Geometry check sheet. Reference: the model listing, model coordinates, mm. Face numbers are marked on the shaded views. A direction names the side the tool comes from. Round coordinates to 2 decimals unless told otherwise and drop trailing zeros. Order: outer loops, then holes, each group sorted by start corner. A loop starts at its lowest first (then second) coordinate and runs counter-clockwise, first axis right, second up. Notation, with made-up numbers: (3.5, -34.5) - (57.5, -34.5) arc R24 ccw to (57.5, 0.5) - close; hole circle Ø10 at (8, -0.75). An arc over 180 degrees is marked (long way). One line per question, with ' | ' between items. Start each with the question number.
Q1. Material ranges on line 1 along Z through (x, y) = (15, 24); line 2 along Y through (x, z) = (16.5, -5); line 3 along X through (y, z) = (4.75, -10), recorded low to high.
Q2. Sectioned sample at C-C, the plane z = -10. Enter the section's corners in (x, y).
Q3. Mould release check, pull along Y, two halves, no side actions. Record for the marked faces 1, 2 and 3: +Y half, -Y half, draft (parallel to the pull), parting line (faces both ways), or undercut.
Q4. Gauge pin test, flat ends, axial feed: P1, Ø8, axis at y = 24.5, z = 13, coming from the -X side; P2, Ø6, axis at x = 16, y = 12, coming from the -Z side; P3, Ø12, axis at x = 8, y = 9.5, coming from the -Z side. Record the tip position at first contact, or that the pin passes through.
Q5. Tool access check on the marked faces 4 and 5. Record the directions out of +Z, -Z, +X, -X, +Y, -Y that give a thin tool (end or side, any length) a straight path to the whole face; none if there is none.
Q6. Sectioned sample at D-D, the plane z = 15.5. Enter the section's corners in (x, y), then the cut area to 3 significant figures.
Q7. Sectioned sample at B-B, the plane z = 35. Enter the section's corners in (x, y), then the cut area to 3 significant figures.
Q8. Sectioned sample at A-A, the plane x = 15. Give the number of separate pieces and of enclosed holes in the cut face, then the cut area to 3 significant figures.
```python
from build123d import *

# Parameters (mm, degrees)
SKETCH3_W            = 30
SKETCH3_H            = 30
BOSS_EXTRUDE1_DEPTH  = 40
CUT_EXTRUDE1_DEPTH   = 10
SKETCH5_R            = 3.58
CUT_EXTRUDE2_DEPTH   = 5
CUT_EXTRUDE4_START   = -40
CUT_EXTRUDE4_DEPTH   = 99.309518948
MIRROR5_START        = -40
MIRROR5_COPY_1_DEPTH = 99.309518948
SKETCH9_R            = 1.75
BOSS_EXTRUDE2_DEPTH  = 30
CUT_EXTRUDE5_DEPTH   = 30
SKETCH11_W           = 20
SKETCH11_H           = 12.2
CUT_EXTRUDE6_DEPTH   = 44.5
SKETCH15_R           = 1.75
CUT_EXTRUDE8_DEPTH   = 25


with BuildPart() as part:
    # Sketch3 → Boss-Extrude1 (new body)
    with BuildSketch(Plane.XY):
        with Locations((15, 15)):
            Rectangle(SKETCH3_W, SKETCH3_H)
    extrude(amount=BOSS_EXTRUDE1_DEPTH)

    # Sketch4 → Cut-Extrude1 (cut)
    with BuildSketch(Plane.XY.offset(40)):
        with BuildLine():
            ThreePointArc((20.75, 15), (17.200429736, 20.312307312), (10.934136008, 19.065863992))
            Line((10.934136008, 19.065863992), (19.065863992, 10.934136008))
            ThreePointArc((19.065863992, 10.934136008), (20.312307312, 12.799570264), (20.75, 15))
        make_face()
        with BuildLine():
            Line((19.065863992, 10.934136008), (10.934136008, 19.065863992))
            ThreePointArc((10.934136008, 19.065863992), (10.934136008, 10.934136008), (19.065863992, 10.934136008))
        make_face()
    extrude(amount=-CUT_EXTRUDE1_DEPTH, mode=Mode.SUBTRACT)

    # Sketch5 → Cut-Extrude2 (cut)
    with BuildSketch(Plane.XZ):
        with Locations(Location((15, 35, 0), (0, 0, 270))):
            Circle(SKETCH5_R)
    extrude(amount=-CUT_EXTRUDE2_DEPTH, mode=Mode.SUBTRACT)

    # Sketch8 → Cut-Extrude4 (cut)
    with BuildSketch(Plane(origin=(0, 0, 0), x_dir=(-1, 0, 0), z_dir=(0, 0, -1)).offset(CUT_EXTRUDE4_START)):
        Polygon((-77.236567429, -51.703622198), (-30, 17.572977849), (-21.526577959, 30), (25.70998947, 99.276600047), (-112.843210625, 193.749734905), (-215.789767524, 42.769512659), align=None)
    cut_extrude4 = extrude(amount=CUT_EXTRUDE4_DEPTH, mode=Mode.SUBTRACT)

    # Mirror4: Cut-Extrude4 across plane
    add(cut_extrude4.mirror(Plane.ZY.offset(-15)), mode=Mode.SUBTRACT)

    # Mirror5: Cut-Extrude4 across plane
    add(cut_extrude4.mirror(Plane(origin=(0, 15, 0), x_dir=(0, 0, 1), z_dir=(0, -1, 0))), mode=Mode.SUBTRACT)

    # Mirror5 copy 1 sketch → Mirror5 copy 1 (cut)
    with BuildSketch(Plane(origin=(30, 30, 0), x_dir=(1, 0, 0), z_dir=(0, 0, -1)).offset(MIRROR5_START)):
        Polygon((-77.236567429, -51.703622198), (-30, 17.572977849), (-21.526577959, 30), (25.70998947, 99.276600047), (-112.843210625, 193.749734905), (-215.789767524, 42.769512659), align=None)
    extrude(amount=MIRROR5_COPY_1_DEPTH, mode=Mode.SUBTRACT)

    # Sketch9 → Boss-Extrude2 (add)
    with BuildSketch(Plane(origin=(0, 0, 0), x_dir=(1, 0, 0), z_dir=(0, 1, 0))):
        with BuildLine():
            Line((5.769230769, 13.846153846), (0, 0))
            Line((0, 0), (30, 0))
            Line((30, 0), (24.924823528, 11.223878236))
            Line((24.924823528, 11.223878236), (22.474176558, 16.643544594))
            ThreePointArc((22.474176558, 16.643544594), (13.348408887, 19.862669355), (5.769230769, 13.846153846))
        make_face()
        with Locations(Location((15, 10, 0), (0, 0, 270))):
            Circle(SKETCH9_R, mode=Mode.SUBTRACT)
    extrude(amount=BOSS_EXTRUDE2_DEPTH)

    # Sketch10 → Cut-Extrude5 (cut)
    with BuildSketch(Plane.XY):
        Polygon((0, 17.572977849), (8.473422041, 30), (0, 30), align=None)
        Polygon((8.473422041, 0), (0, 0), (0, 12.427022151), align=None)
        Polygon((21.526577959, 0), (30, 12.427022151), (30, 0), align=None)
        Polygon((30, 17.572977849), (21.526577959, 30), (30, 30), align=None)
    extrude(amount=-CUT_EXTRUDE5_DEPTH, mode=Mode.SUBTRACT)

    # Sketch11 → Cut-Extrude6 (cut, symmetric)
    with BuildSketch(Plane(origin=(30, 0, 0), x_dir=(0, 0, -1), z_dir=(1, 0, 0))):
        with Locations((10, 15)):
            Rectangle(SKETCH11_W, SKETCH11_H)
    extrude(amount=CUT_EXTRUDE6_DEPTH, both=True, mode=Mode.SUBTRACT)

    # Sketch15 → Cut-Extrude8 (cut)
    with BuildSketch(Plane.XZ.offset(-5)):
        with Locations(Location((15, 35, 0), (0, 0, 270))):
            Circle(SKETCH15_R)
    extrude(amount=-CUT_EXTRUDE8_DEPTH, mode=Mode.SUBTRACT)


solid = part.part
```
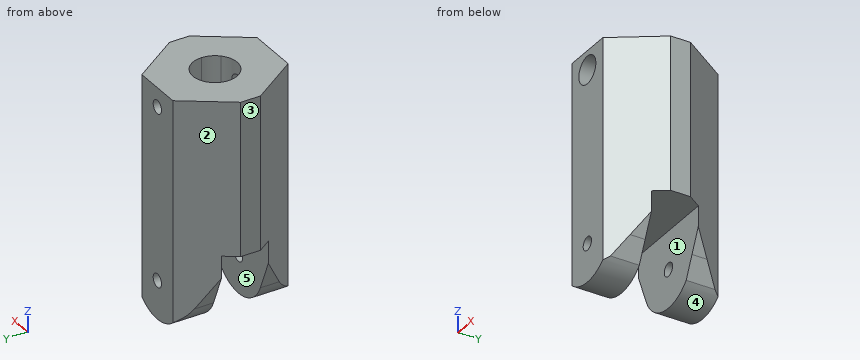
Determined:
1) line 1: z = -20 to -11.75, -8.25 to 33.25, 36.75 to 40 | line 2: y = 0 to 8.9, 21.1 to 30 | line 3: x = 5.23 to 13.25, 16.75 to 24.77
2) outline: (4.17, 6.32) - (8.47, 0) - (13.25, 0) - (13.25, 8.9) - (4.17, 8.9) - close; (4.17, 21.1) - (13.25, 21.1) - (13.25, 30) - (8.47, 30) - (4.17, 23.68) - close; (16.75, 0) - (21.53, 0) - (25.48, 5.8) - (25.48, 8.9) - (16.75, 8.9) - close; (16.75, 21.1) - (25.48, 21.1) - (25.48, 24.2) - (21.53, 30) - (16.75, 30) - close
3) face 1: undercut | face 2: +Y half | face 3: draft
4) P1: stops at x = 2 | P2: stops at z = 0 | P3: stops at z = -19.95
5) face 4: -Z, +Y, -Y | face 5: -Z, +X, -X
6) outline: (0, 12.43) - (8.47, 0) - (21.53, 0) - (30, 12.43) - (30, 17.57) - (21.53, 30) - (8.47, 30) - (0, 17.57) - close | area: 689 mm2
7) outline: (0, 12.43) - (8.47, 0) - (11.42, 0) - (11.42, 5) - (13.25, 5) - (13.25, 9.52) arc R5.75 cw to (13.25, 20.48) - (13.25, 30) - (8.47, 30) - (0, 17.57) - close; (16.75, 5) - (18.58, 5) - (18.58, 0) - (21.53, 0) - (30, 12.43) - (30, 17.57) - (21.53, 30) - (16.75, 30) - (16.75, 20.48) arc R5.75 cw to (16.75, 9.52) - close | area: 502 mm2
8) separate pieces: 5 | enclosed holes: 0 | area: 1,300 mm2
